```python
from build123d import *

# Parameters (mm, degrees)
SKETCH_1_R               = 40
SKETCH_1_R_2             = 29
EXTRUDE_1_DEPTH          = 4.5
SKETCH_2_R               = 37.8
SKETCH_2_R_2             = 33.5
EXTRUDE_2_DEPTH          = 10
FILLET_1_R               = 1
FILLET_2_R               = 3
SKETCH_3_R               = 1.6
CUT_EXTRUDE_1_DEPTH      = 41
CUT_EXTRUDE_1_DEPTH_BACK = 41.0000001
SKETCH_4_R               = 1.6
CUT_EXTRUDE_2_DEPTH      = 41
CUT_EXTRUDE_2_DEPTH_BACK = 41


with BuildPart() as part:
    # 草图1 → 凸台-拉伸1 (new body)
    with BuildSketch(Plane(origin=(0, 0, 0), x_dir=(1, 0, 0), z_dir=(0, 1, 0))):
        Circle(SKETCH_1_R)
        Circle(SKETCH_1_R_2, mode=Mode.SUBTRACT)
    extrude(amount=EXTRUDE_1_DEPTH)

    # 草图2 → 凸台-拉伸2 (add)
    with BuildSketch(Plane.XZ):
        Circle(SKETCH_2_R)
        Circle(SKETCH_2_R_2, mode=Mode.SUBTRACT)
    extrude(amount=EXTRUDE_2_DEPTH)

    # 圆角1
    fillet_1_edges = [part.edges().sort_by_distance(p)[0] for p in [
        (-37.8, -10, 0),
        (-33.5, -10, 0),
    ]]
    fillet(fillet_1_edges, radius=FILLET_1_R)

    # 圆角2
    fillet_2_edges = [part.edges().sort_by_distance(p)[0] for p in [
        (-40, 4.5, 0),
    ]]
    fillet(fillet_2_edges, radius=FILLET_2_R)

    # 草图3 → 切除-拉伸1 (cut, two sides)
    with BuildSketch(Plane(origin=(0, 0, 0), x_dir=(0, 0, -1), z_dir=(1, 0, 0))) as cut_extrude_1_sk:
        with Locations((0, -4)):
            Circle(SKETCH_3_R)
    extrude(amount=CUT_EXTRUDE_1_DEPTH, mode=Mode.SUBTRACT)
    extrude(cut_extrude_1_sk.sketch, amount=-CUT_EXTRUDE_1_DEPTH_BACK, mode=Mode.SUBTRACT)

    # 草图4 → 切除-拉伸2 (cut, two sides)
    with BuildSketch(Plane.XY) as cut_extrude_2_sk:
        with Locations((0, -4)):
            Circle(SKETCH_4_R)
    extrude(amount=CUT_EXTRUDE_2_DEPTH, mode=Mode.SUBTRACT)
    extrude(cut_extrude_2_sk.sketch, amount=-CUT_EXTRUDE_2_DEPTH_BACK, mode=Mode.SUBTRACT)


solid = part.part
```
Verification items for the finished model (mm, model axes). A direction names the side the tool comes from. Give positions to 0.01 mm unless a question says otherwise; leave off trailing zeros. Order: outer loops, then holes, each group sorted by start corner. A loop starts at its lowest first (then second) coordinate and runs counter-clockwise, first axis right, second up. Notation, with made-up numbers: (51, 70.25) - (94, 70.25) arc R24 ccw to (94, 84.25) - close; hole circle Ø5 at (62, 28). An arc over 180 degrees is marked (long way). Answer as CSV lines item,"result". Start each with the question number.
Item 1: Mould release check, pull along Y, two halves, no side actions. Record for faces 1 (the face through (-22.1, 4.5, 19.01)), 2 (the face through (-0.208, -2.414, -35.6)), 3 (the face through (35, 0, 15)): released by +Y, released by -Y, zero draft, split by the parting line, or undercut.
Item 2: Section check C-C, the plane y = -4. Record the boundary of the cut face in (x, z).
Item 3: Gauge pin test, flat ends, axial feed: pin 1 (6 mm diameter, centred on y = -7.5, z = -29.5, fed in from +X); pin 2 (10 mm diameter, centred on x = -32, z = -30.5, fed in from -Y); pin 3 (3.5 mm diameter, centred on y = -4, z = 0, fed in from +X). Record the tip position at first contact, or that the pin passes through.
Item 4: Section check A-A, the plane z = 0. State how many separate pieces and enclosed holes the cut face has, plus the area to 3 significant figures.
Item 5: Material ranges on L1, parallel to Z at x = 0, y = -2; L2, parallel to Y at x = 36.9, z = 0, recorded low to high.
Item 6: Access from +Z, -Z, +X, -X, +Y, -Y to the whole of each face (thin tool, end or side, straight path). Record for faces 4 (the face through (-10.1, 0, -27.5)), 5 (the face through (-35.6, -2.414, 0.208)).
Filled in:
1,face 1,"released by +Y"
1,face 2,"undercut"
1,face 3,"released by -Y"
2,outline,"(-37.77, -1.6) arc R37.8 ccw to (-1.6, -37.77) - (-1.6, -33.46) arc R33.5 cw to (-33.46, -1.6) - close; (-37.77, 1.6) - (-33.46, 1.6) arc R33.5 cw to (-1.6, 33.46) - (-1.6, 37.77) arc R37.8 ccw to start; (1.6, -37.77) arc R37.8 ccw to (37.77, -1.6) - (33.46, -1.6) arc R33.5 cw to (1.6, -33.46) - close; (1.6, 33.46) arc R33.5 cw to (33.46, 1.6) - (37.77, 1.6) arc R37.8 ccw to (1.6, 37.77) - close"
3,pin 1,"x = 26.96"
3,pin 2,"y = 0"
3,pin 3,"x = 37.8"
4,separate pieces,"4"
4,enclosed holes,"0"
4,area,"153 mm^2"
5,L1,"-37.8 to -33.5, 33.5 to 37.8"
5,L2,"-9.99 to -5.6, -2.4 to 4.5"
6,face 4,"-Y"
6,face 5,"+X, -X"
